Model file for the job. Use its own axes, mm. Round coordinates to 2 decimals unless told otherwise and drop trailing zeros. Use one line per item in the form item = value.
from build123d import *

# Parameters (mm, degrees)
SKETCH1_W           = 101.6
SKETCH1_H           = 63.5
BOSS_EXTRUDE1_DEPTH = 3.175
SKETCH2_R           = 0.79375
CUT_EXTRUDE1_DEPTH  = 6.35
SKETCH3_R           = 0.79375
CUT_EXTRUDE2_DEPTH  = 6.35
SKETCH4_R           = 1.19761
CUT_EXTRUDE3_DEPTH  = 4.175


with BuildPart() as part:
    # Sketch1 → Boss-Extrude1 (new body)
    with BuildSketch(Plane(origin=(0, 0, 0), x_dir=(1, 0, 0), z_dir=(0, 1, 0))):
        with Locations((8.595554542, -11.095875723)):
            Rectangle(SKETCH1_W, SKETCH1_H)
    extrude(amount=BOSS_EXTRUDE1_DEPTH)

    # Sketch2 → Cut-Extrude1 (cut)
    with BuildSketch(Plane.XY.offset(42.845875723)):
        with Locations((-40.616945458, 1.5875)):
            Circle(SKETCH2_R)
        with Locations((57.808054542, 1.5875)):
            Circle(SKETCH2_R)
    extrude(amount=-CUT_EXTRUDE1_DEPTH, mode=Mode.SUBTRACT)

    # Sketch3 → Cut-Extrude2 (cut)
    with BuildSketch(Plane(origin=(0, 0, -20.654124277), x_dir=(-1, 0, 0), z_dir=(0, 0, -1))):
        with Locations(Location((-57.808054542, 1.5875, 0), (0, 0, 180))):  # turned: the seam where the file's is
            Circle(SKETCH3_R)
        with Locations(Location((40.616945458, 1.5875, 0), (0, 0, 180))):  # turned: the seam where the file's is
            Circle(SKETCH3_R)
    extrude(amount=-CUT_EXTRUDE2_DEPTH, mode=Mode.SUBTRACT)

    # Sketch4 → Cut-Extrude3 (cut, through all)
    with BuildSketch(Plane(origin=(0, 3.175, 0), x_dir=(1, 0, 0), z_dir=(0, 1, 0))):
        with Locations(Location((-20.868445458, 13.034124277, 0), (0, 0, 270))):  # turned: the seam where the file's is
            Circle(SKETCH4_R)
        with Locations(Location((-22.138445458, -35.225875723, 0), (0, 0, 270))):  # turned: the seam where the file's is
            Circle(SKETCH4_R)
        with Locations(Location((29.931554542, -2.205875723, 0), (0, 0, 270))):  # turned: the seam where the file's is
            Circle(SKETCH4_R)
        with Locations(Location((29.931554542, -30.145875723, 0), (0, 0, 270))):  # turned: the seam where the file's is
            Circle(SKETCH4_R)
    extrude(amount=-CUT_EXTRUDE3_DEPTH, mode=Mode.SUBTRACT)


solid = part.part
1. Pull direction Z, two halves, no side cores. Call faces 1 (the cylindrical face through (-22.04, 1.61, -13.29)), 2 (the flat face through (8, 2, -20.654)), 3 (the flat face through (8, 2, 42.846)): +Z half, -Z half, draft (parallel to the pull), parting line (faces both ways), or undercut.
Geometry check:
face_1 = undercut
face_2 = -Z half
face_3 = +Z half
2. Wall check: probe 1 along Z at (x, y) = (29.5, 0.2). Give the ranges that are in metal, low to high.
Geometry check:
probe_1 = -20.65 to 1.09, 3.32 to 29.03, 31.26 to 42.85
3. Flat gauge pins, fed straight in: pin 1 (1.5 mm diameter, centred on x = -32, z = 24.5, fed in from -Y); pin 2 (1.4 mm diameter, centred on x = -40.62, y = 1.59, fed in from -Z); pin 3 (1.4 mm diameter, centred on x = -40.62, y = 1.59, fed in from +Z); pin 4 (2 mm diameter, centred on x = -22.14, z = 35.23, fed in from +Y). Where does each tip first touch, or does it go through?
Geometry check:
pin_1 = 0
pin_2 = -14.3
pin_3 = 36.5
pin_4 = through
